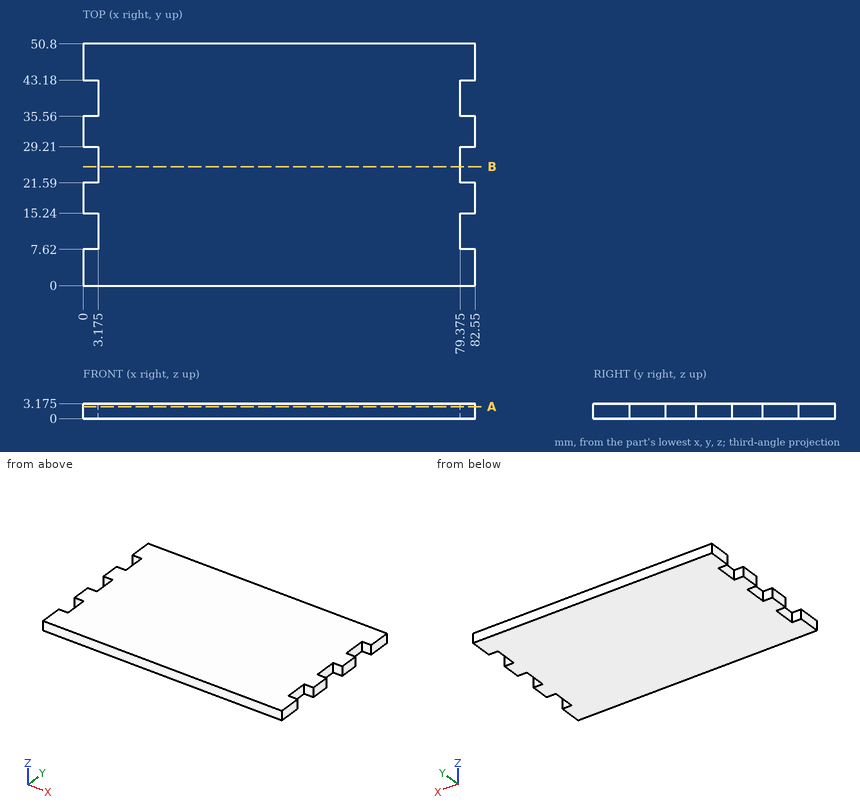
Can you work these out from the drawing? Everything is in mm from the part's minimum corner. Round coordinates to 2 decimals unless told otherwise and drop trailing zeros. Write each loop counter-clockwise with the first axis right and the second up, starting at its lowest first coordinate (ties: lowest second). Pieces come first, ordered by that corner, then holes. Notation, with made-up numbers: M 32,77.25 L 64,77.25 A22 cw 64,103.25 Z; hole C 16,-27 d4. An arc over 180 degrees is marked long. Use a Markdown table: item, result.
Item 1: If I drill on line 1 along X through (y, z) = (39, 1.7) (3 decimals), over which ranges is the centre line in solid material (lowest first)? Write a range as [from, to].
Found:
| item | result |
|---|---|
| line 1 | x = [3.175, 79.375] |
Item 2: I want a section at A-A (z = 2.5). List the corners of the cut face in (x, y) for me (3 decimals), and give its area (3 significant figures).
Found:
| item | result |
|---|---|
| outline | M 0,0 L 82.55,0 L 82.55,7.62 L 79.375,7.62 L 79.375,15.24 L 82.55,15.24 L 82.55,21.59 L 79.375,21.59 L 79.375,29.21 L 82.55,29.21 L 82.55,35.56 L 79.375,35.56 L 79.375,43.18 L 82.55,43.18 L 82.55,50.8 L 0,50.8 L 0,43.18 L 3.175,43.18 L 3.175,35.56 L 0,35.56 L 0,29.21 L 3.175,29.21 L 3.175,21.59 L 0,21.59 L 0,15.24 L 3.175,15.24 L 3.175,7.62 L 0,7.62 Z |
| area | 4,050 mm2 |
Item 3: For pin 1 Ø1.6 at (y, z) = (12.5, 2) entering from -X (3 decimals); pin 2 Ø1 at (y, z) = (26, 2.5) entering from +X (3 decimals), each with a flat end and sliding along its axis, tell me the tip position at first contact or that it passes through.
Found:
| item | result |
|---|---|
| pin 1 | stops at x = 3.175 |
| pin 2 | stops at x = 79.375 |
Item 4: I want a section at B-B (y = 25). List the corners of the cut face in (x, z) for me (3 decimals).
Found:
| item | result |
|---|---|
| outline | M 3.175,0 L 79.375,0 L 79.375,3.175 L 3.175,3.175 Z |
